Model file for the job. Use its own axes, mm. A direction names the side the tool comes from. Give positions to 0.01 mm unless a question says otherwise; leave off trailing zeros. Order: outer loops, then holes, each group sorted by start corner. A loop starts at its lowest first (then second) coordinate and runs counter-clockwise, first axis right, second up. Notation, with made-up numbers: M 14,67.25 L 47,67.25 A11 cw 47,87.25 Z; hole C 31,45.25 d5. An arc over 180 degrees is marked long. Return JSON: item names as keys, results as strings. Group by question number.
1. 3-axis set-ups, long thin cutter, end or side, ignore diameter. For faces 4 (the face through (19, 33.528, 6)), 5 (the face through (74.478, 51.947, 7.513)), 6 (the face through (18, 44.323, 6)): which of +Z, -Z, +X, -X, +Y, -Y reach the whole face in a straight line?
2. Wall check: probe 1 along X at (y, z) = (19, 1.75) (3 decimals); probe 2 along Y at (x, z) = (70, 12) (3 decimals); probe 3 along Y at (x, z) = (50, 10.25) (3 decimals). Give the ranges that are in metal, low to high. Write a range as [from, to].
3. Pin check, flat tips, straight feed: pin 1 (7 mm diameter, centred on y = 5.5, z = 6.5, fed in from -X) (3 decimals); pin 2 (2 mm diameter, centred on x = 75.565, y = 19.05, fed in from +Z); pin 3 (3.5 mm diameter, centred on x = 18.415, z = 7.62, fed in from +Y); pin 4 (1 mm diameter, centred on x = 45, z = 8, fed in from +Y). Stop position of each tip, or through.
4. Two-plate mould, pull along X, no slides. Class faces 1 (the face through (34.925, 17, 8)), 2 (the face through (10.774, 90.164, 7.513)), 3 (the face through (17.125, 39.001, 7.085)): released by +X, released by -X, zero draft, split by the parting line, or undercut.
5. Slice it at B-B on x = 58. List the corners of the cut face in (y, z) (3 decimals), then the cut area to 3 significant figures.
from build123d import *

# Parameters (mm, degrees)
BOSS_EXTRUDE1_DEPTH = 2.54
BOSS_EXTRUDE2_DEPTH = 12.7
BOSS_EXTRUDE3_DEPTH = 7.62
SKETCH5_R           = 1.397
CUT_EXTRUDE1_DEPTH  = 104.117521798
SKETCH6_R           = 4.445
BOSS_EXTRUDE4_DEPTH = 12.7
SKETCH7_R           = 6.35
CUT_EXTRUDE2_DEPTH  = 130.279824509
SKETCH8_R           = 1.397
CUT_EXTRUDE3_DEPTH  = 130.279824509
BOSS_EXTRUDE5_DEPTH = 7.62
SKETCH10_R          = 1.397
CUT_EXTRUDE4_DEPTH  = 122.944757421


with BuildPart() as part:
    # Sketch2 → Boss-Extrude1 (new body)
    with BuildSketch(Plane.XY):
        with BuildLine():
            Line((34.925, 0), (90.805, 0))
            ThreePointArc((90.805, 0), (65.321718823, 63.07631152), (3.175, 90.749476032))
            Line((3.175, 90.749476032), (3.175, 33.528))
            Line((3.175, 33.528), (34.925, 33.528))
            Line((34.925, 33.528), (34.925, 0))
        make_face()
    extrude(amount=BOSS_EXTRUDE1_DEPTH)

    # Sketch3 → Boss-Extrude2 (add)
    with BuildSketch(Plane.XY.offset(2.54)):
        with BuildLine():
            Line((34.925, 33.528), (34.925, 0))
            Line((34.925, 0), (90.805, 0))
            ThreePointArc((90.805, 0), (65.321718823, 63.07631152), (3.175, 90.749476032))
            Line((3.175, 90.749476032), (3.175, 33.528))
            Line((3.175, 33.528), (34.925, 33.528))
        make_face()
        with BuildLine():
            Line((6.35, 36.703), (38.1, 36.703))
            Line((38.1, 36.703), (38.1, 3.175))
            Line((38.1, 3.175), (87.572462995, 3.175))
            ThreePointArc((87.572462995, 3.175), (63.077762451, 60.829374353), (6.35, 87.399624713))
            Line((6.35, 87.399624713), (6.35, 36.703))
        make_face(mode=Mode.SUBTRACT)
    extrude(amount=BOSS_EXTRUDE2_DEPTH)

    # Sketch4 → Boss-Extrude3 (add)
    with BuildSketch(Plane(origin=(0, 36.703, 0), x_dir=(1, 0, 0), z_dir=(0, 1, 0))):
        with BuildLine():
            Line((14.605, -7.62), (14.605, 0))
            Line((14.605, 0), (22.225, 0))
            Line((22.225, 0), (22.225, -7.62))
            ThreePointArc((22.225, -7.62), (18.415, -11.43), (14.605, -7.62))
        make_face()
    extrude(amount=BOSS_EXTRUDE3_DEPTH)

    # Sketch5 → Cut-Extrude1 (cut, through all)
    with BuildSketch(Plane(origin=(0, 44.323, 0), x_dir=(1, 0, 0), z_dir=(0, 1, 0))):
        with Locations(Location((18.415, -7.62, 0), (0, 0, 180))):
            Circle(SKETCH5_R)
    extrude(amount=-CUT_EXTRUDE1_DEPTH, mode=Mode.SUBTRACT)

    # Sketch6 → Boss-Extrude4 (add)
    with BuildSketch(Plane.XY.offset(2.54)):
        with Locations((43.815, 44.45)):
            Circle(SKETCH6_R)
        with Locations((43.815, 69.85)):
            Circle(SKETCH6_R)
        with Locations((50.165, 19.05)):
            Circle(SKETCH6_R)
        with Locations((75.565, 19.05)):
            Circle(SKETCH6_R)
        with Locations((69.215, 44.45)):
            Circle(SKETCH6_R)
    extrude(amount=BOSS_EXTRUDE4_DEPTH)

    # Sketch7 → Cut-Extrude2 (cut, through all)
    with BuildSketch(Plane.XY.offset(15.24)):
        with Locations((23.540776994, 85.726552587)):
            Circle(SKETCH7_R)
    extrude(amount=-CUT_EXTRUDE2_DEPTH, mode=Mode.SUBTRACT)

    # Sketch8 → Cut-Extrude3 (cut, through all)
    with BuildSketch(Plane.XY.offset(15.24)):
        with Locations((43.815, 69.85)):
            Circle(SKETCH8_R)
        with Locations((43.815, 44.45)):
            Circle(SKETCH8_R)
        with Locations((69.215, 44.45)):
            Circle(SKETCH8_R)
        with Locations((75.565, 19.05)):
            Circle(SKETCH8_R)
        with Locations((50.165, 19.05)):
            Circle(SKETCH8_R)
    extrude(amount=-CUT_EXTRUDE3_DEPTH, mode=Mode.SUBTRACT)

    # Sketch9 → Boss-Extrude5 (add)
    with BuildSketch(Plane(origin=(0, 3.175, 0), x_dir=(1, 0, 0), z_dir=(0, 1, 0))):
        with BuildLine():
            Line((66.646231497, -8.89), (66.646231497, -2.54))
            Line((66.646231497, -2.54), (59.026231497, -2.54))
            Line((59.026231497, -2.54), (59.026231497, -8.89))
            ThreePointArc((59.026231497, -8.89), (62.836231497, -12.7), (66.646231497, -8.89))
        make_face()
    extrude(amount=BOSS_EXTRUDE5_DEPTH)

    # Sketch10 → Cut-Extrude4 (cut, through all)
    with BuildSketch(Plane(origin=(0, 10.795, 0), x_dir=(1, 0, 0), z_dir=(0, 1, 0))):
        with Locations(Location((62.836231497, -8.89, 0), (0, 0, 270))):
            Circle(SKETCH10_R)
    extrude(amount=-CUT_EXTRUDE4_DEPTH, mode=Mode.SUBTRACT)


solid = part.part
Result:
{
 "1": {"face 4": "+Z, -Z, -X, -Y", "face 5": "+Z, -Z, +X, +Y", "face 6": "+Z"},
 "2": {"probe 1": "x = [34.925, 48.769], [51.561, 74.169], [76.961, 88.795]", "probe 2": "y = [0, 3.175], [40.075, 43.294], [45.606, 48.825], [52.716, 57.841]", "probe 3": "y = [0, 3.175], [14.608, 17.663], [20.437, 23.492], [71.965, 75.799]"},
 "3": {"pin 1": "stops at x = 34.925", "pin 2": "passes through", "pin 3": "stops at y = 89.26", "pin 4": "stops at y = 79.15"},
 "4": {"face 1": "released by -X", "face 2": "released by +X", "face 3": "undercut"},
 "5": {"outline": "M 0,0 L 69.868,0 L 69.868,15.24 L 65.689,15.24 L 65.689,2.54 L 3.175,2.54 L 3.175,15.24 L 0,15.24 Z", "area": "271 mm2"}
}
